from build123d import *

# Parameters (mm, degrees)
F0_R           = 5.5
F1_DEPTH       = 3
F3_D           = 3.2
F3_DEPTH       = 12
F3_CSINK_D     = 7.75
F3_CSINK_ANGLE = 90
F3_TIP         = 0.9613769904


# Not quite as in the source:
# - a fillet or chamfer that OpenCascade refuses, or shapes differently, is made with other operations: its cross-section is extruded or revolved along the edge and cut away or added


with BuildPart() as f1:
    # F0 (on Top) → F1 (new body)
    with BuildSketch(Plane.XY):
        with Locations((-42.9622493684, 14.7040970623)):
            Circle(F0_R)
    extrude(amount=F1_DEPTH)

    # F3
    with Locations(Plane.XY.offset(3)):
        with Locations((-42.9622493684, 14.7040970623)):
            CounterSinkHole(F3_D / 2, F3_CSINK_D / 2, depth=F3_DEPTH, counter_sink_angle=F3_CSINK_ANGLE)
            with Locations((0, 0, -(F3_DEPTH + F3_TIP / 2))):  # 118° drill point
                Cone(0, F3_D / 2, F3_TIP, mode=Mode.SUBTRACT)

    # F4: chamfer of 2 on 1 edges, made by hand

    # F4_s1 → F4_t2 (revolve, cut)
    with BuildSketch(Plane.XZ.offset(-14.7040970623)):
        Polygon((-37.4622493684, 1), (-39.4622493684, 3), (-37.4622493684, 3), align=None)
    revolve(axis=Axis((-42.9622493684, 14.7040970623, 3), (0, 0, 1)), mode=Mode.SUBTRACT)


solid = f1.part
Could you check a few things on this model? Use its own coordinates, in mm. Round coordinates to 2 decimals unless told otherwise and drop trailing zeros. Order: outer loops, then holes, each group sorted by start corner. A loop starts at its lowest first (then second) coordinate and runs counter-clockwise, first axis right, second up. Notation, with made-up numbers: M 81.25,63.5 L 85.25,63.5 A21 cw 85.25,72.5 Z; hole C 12,-39 d5. An arc over 180 degrees is marked long. One line per item, written item: value.
(1) Imagine slicing it at B-B (z = 2.55). Write out the boundary of the cut face in (x, y) (3 decimals).
Ans:
outline: C -42.962,14.704 d7.9; hole C -42.962,14.704 d6.85
(2) Imagine slicing it at A-A (z = 1.85). Write out the boundary of the cut face in (x, y) (3 decimals).
Ans:
outline: C -42.962,14.704 d9.3; hole C -42.962,14.704 d5.45
(3) If we mould it in two halves opening along Y, with no side actions, what happens to faces 1 (the cylindrical face through (-43.701, 13.285, 0.357)), 2 (the conical face through (-43.8, 11, 2.7)), 3 (the flat face through (-44.3, 16, 0))? For each: released by +Y, released by -Y, zero draft, split by the parting line, or undercut.
Ans:
face 1: undercut
face 2: split by the parting line
face 3: zero draft
(4) I need wall thicknesses on line 1 along X through (y, z) = (15.5, 0.95); line 2 along Y through (x, z) = (-44, 2.6); line 3 along X through (y, z) = (13.75, 1.75). Which ranges of each line are inside material? Lowest first, please. Write a range as from..to.
Ans:
line 1: x = -48.4..-44.6, -41.32..-37.52
line 2: y = 10.94..11.39, 18.02..18.46
line 3: x = -47.62..-45.41, -40.52..-38.31
(5) I'm going to push flat-ended pins straight in: P1, Ø1.5, axis at y = 18, z = 1, coming from the +X side; P2, Ø2.5, axis at x = -42.96, y = 14.7, coming from the +Z side. Where does each tip first touch, or does it pass through?
Ans:
P1: stops at x = -38.09
P2: passes through
